Design review of the part built by this model. Coordinates are the model's own, in mm. Face numbers are marked on the shaded views. Coordinates: 2 decimals unless noted, no trailing zeros. Loops run counter-clockwise (first coordinate to the right, second up) from the corner with the lowest first, then second, coordinate; pieces in that order, holes last. Notation, with made-up numbers: (34.25, 73) - (69.25, 73) arc R24 ccw to (69.25, 83) - close; hole circle Ø5 at (48, 74.5). An arc over 180 degrees is marked (long way). One line per question, with ' | ' between items.
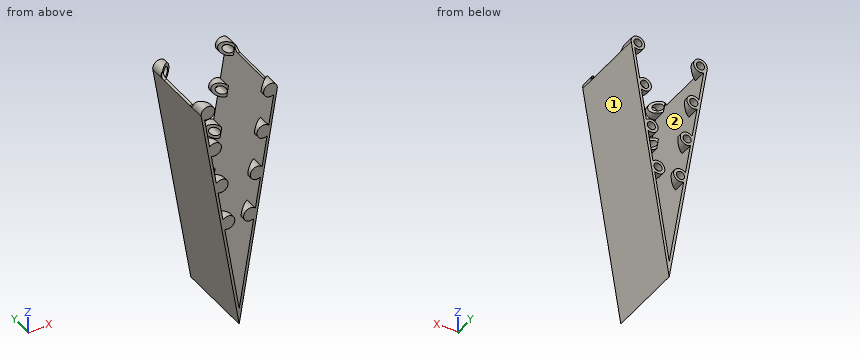
from build123d import *

# Parameters (mm, degrees)
BOSS_EXTRUDE1_DEPTH            = 30
SKETCH2_R                      = 2.6
SKETCH2_R_2                    = 1.55
BOSS_EXTRUDE3_DEPTH            = 5
CUT_EXTRUDE1_REACH             = 100.017
CUT_EXTRUDE1_DIRECTION_2_DEPTH = 99.016911981
CUT_EXTRUDE2_REACH             = 100.017
CUT_EXTRUDE2_DIRECTION_2_DEPTH = 99.016911981
FILLET1_R                      = 2
SKETCH6_R                      = 2.6
BOSS_EXTRUDE4_DEPTH            = 1


with BuildPart() as part:
    # Sketch1 → Boss-Extrude1 (new body)
    with BuildSketch(Plane(origin=(0, 0, 0), x_dir=(1, 0, 0), z_dir=(0, 1, 0))):
        Polygon((-13.5, 0), (0, 83.718518379), (13.5, 0), (14.487246657, 0.15919811), (0, 90), (-14.487246657, 0.15919811), align=None)
    extrude(amount=BOSS_EXTRUDE1_DEPTH)

    # Sketch2 → Boss-Extrude3 (add)
    # profile 1 of 8: a face of its own
    with BuildSketch(Plane(origin=(0, 0, 0), x_dir=(1, 0, 0), z_dir=(0, 1, 0))):
        with Locations((11.920405349, -0.254716975)):
            Circle(SKETCH2_R)
        with Locations(Location((11.920405349, -0.254716975, 0), (0, 0, 270))):
            Circle(SKETCH2_R_2, mode=Mode.SUBTRACT)
    # profile 2 of 8: a face of its own
    with BuildSketch(Plane(origin=(0, 0, 0), x_dir=(1, 0, 0), z_dir=(0, 1, 0))):
        with Locations((9.373235594, 15.541229537)):
            Circle(SKETCH2_R)
        with Locations(Location((9.373235594, 15.541229537, 0), (0, 0, 270))):
            Circle(SKETCH2_R_2, mode=Mode.SUBTRACT)
    # profile 3 of 8: a face of its own
    with BuildSketch(Plane(origin=(0, 0, 0), x_dir=(1, 0, 0), z_dir=(0, 1, 0))):
        with Locations((6.826065839, 31.33717605)):
            Circle(SKETCH2_R)
        with Locations(Location((6.826065839, 31.33717605, 0), (0, 0, 270))):
            Circle(SKETCH2_R_2, mode=Mode.SUBTRACT)
    # profile 4 of 8: a face of its own
    with BuildSketch(Plane(origin=(0, 0, 0), x_dir=(1, 0, 0), z_dir=(0, 1, 0))):
        with Locations((4.278896085, 47.133122563)):
            Circle(SKETCH2_R)
        with Locations(Location((4.278896085, 47.133122563, 0), (0, 0, 270))):
            Circle(SKETCH2_R_2, mode=Mode.SUBTRACT)
    # profile 5 of 8: a face of its own
    with BuildSketch(Plane(origin=(0, 0, 0), x_dir=(1, 0, 0), z_dir=(0, 1, 0))):
        with Locations((-4.278896085, 47.133122563)):
            Circle(SKETCH2_R)
        with Locations(Location((-4.278896085, 47.133122563, 0), (0, 0, 90))):
            Circle(SKETCH2_R_2, mode=Mode.SUBTRACT)
    # profile 6 of 8: a face of its own
    with BuildSketch(Plane(origin=(0, 0, 0), x_dir=(1, 0, 0), z_dir=(0, 1, 0))):
        with Locations((-6.826065839, 31.33717605)):
            Circle(SKETCH2_R)
        with Locations(Location((-6.826065839, 31.33717605, 0), (0, 0, 90))):
            Circle(SKETCH2_R_2, mode=Mode.SUBTRACT)
    # profile 7 of 8: a face of its own
    with BuildSketch(Plane(origin=(0, 0, 0), x_dir=(1, 0, 0), z_dir=(0, 1, 0))):
        with Locations((-9.373235594, 15.541229537)):
            Circle(SKETCH2_R)
        with Locations(Location((-9.373235594, 15.541229537, 0), (0, 0, 90))):
            Circle(SKETCH2_R_2, mode=Mode.SUBTRACT)
    # profile 8 of 8: a face of its own
    with BuildSketch(Plane(origin=(0, 0, 0), x_dir=(1, 0, 0), z_dir=(0, 1, 0))):
        with Locations((-11.920405349, -0.254716975)):
            Circle(SKETCH2_R)
        with Locations(Location((-11.920405349, -0.254716975, 0), (0, 0, 90))):
            Circle(SKETCH2_R_2, mode=Mode.SUBTRACT)
    boss_extrude3 = extrude(amount=BOSS_EXTRUDE3_DEPTH)

    # Cut-Extrude1: up to this face of the body (flat: up to its plane)
    cut_extrude1_end = Plane(part.part.faces().sort_by_distance((-6.68152525, 15.362665762, -42.28389657))[0])
    # Sketch4 → Cut-Extrude1 (cut, up to the picked face)
    with BuildSketch(Plane(origin=(0.342144515, 0, 2.121765321), x_dir=(0.9872466570606503, 0, -0.1591981096702188), z_dir=(0.1591981096702188, 0, 0.9872466570606503)), mode=Mode.PRIVATE) as cut_extrude1_sk1:
        Polygon((13.32782987, 5), (9.12782987, 5), (9.12782987, 1.475781549), align=None)
    cut_extrude1_tool1 = split(extrude(cut_extrude1_sk1.sketch, amount=-CUT_EXTRUDE1_REACH, mode=Mode.PRIVATE), bisect_by=cut_extrude1_end, keep=Keep.BOTH, mode=Mode.PRIVATE)
    cut_extrude1 = cut_extrude1_tool1.solids().sort_by(Axis((10.735709, 3.825261, 0.445755), (-0.1591981096702188, 0, -0.9872466570606503)))[0]
    add(cut_extrude1, mode=Mode.SUBTRACT)

    # Sketch4 → Cut-Extrude1 direction 2 (cut)
    with BuildSketch(Plane(origin=(0.342144515, 0, 2.121765321), x_dir=(0.9872466570606503, 0, -0.1591981096702188), z_dir=(0.1591981096702188, 0, 0.9872466570606503))):
        Polygon((13.32782987, 5), (9.12782987, 5), (9.12782987, 1.475781549), align=None)
    cut_extrude1_direction_2 = extrude(amount=CUT_EXTRUDE1_DIRECTION_2_DEPTH, mode=Mode.SUBTRACT)

    # Cut-Extrude2: up to this face of the body (flat: up to its plane)
    cut_extrude2_end = Plane(part.part.faces().sort_by_distance((6.68152525, 15.362665762, -42.28389657))[0])
    # Sketch5 → Cut-Extrude2 (cut, up to the picked face)
    with BuildSketch(Plane(origin=(-0.342144515, 0, 2.121765321), x_dir=(0.9872466570606502, 0, 0.15919810967021986), z_dir=(-0.15919810967021986, 0, 0.9872466570606502)), mode=Mode.PRIVATE) as cut_extrude2_sk1:
        Polygon((-9.12782987, 5), (-9.12782987, 1.475781549), (-13.32782987, 5), align=None)
    cut_extrude2_tool1 = split(extrude(cut_extrude2_sk1.sketch, amount=-CUT_EXTRUDE2_REACH, mode=Mode.PRIVATE), bisect_by=cut_extrude2_end, keep=Keep.BOTH, mode=Mode.PRIVATE)
    cut_extrude2 = cut_extrude2_tool1.solids().sort_by(Axis((-10.735709, 3.825261, 0.445755), (0.15919810967021986, 0, -0.9872466570606502)))[0]
    add(cut_extrude2, mode=Mode.SUBTRACT)

    # Sketch5 → Cut-Extrude2 direction 2 (cut)
    with BuildSketch(Plane(origin=(-0.342144515, 0, 2.121765321), x_dir=(0.9872466570606502, 0, 0.15919810967021986), z_dir=(-0.15919810967021986, 0, 0.9872466570606502))):
        Polygon((-9.12782987, 5), (-9.12782987, 1.475781549), (-13.32782987, 5), align=None)
    cut_extrude2_direction_2 = extrude(amount=CUT_EXTRUDE2_DIRECTION_2_DEPTH, mode=Mode.SUBTRACT)

    # Mirror2: Boss-Extrude3, Cut-Extrude1, Cut-Extrude1 direction 2, Cut-Extrude2, Cut-Extrude2 direction 2 across plane
    add(boss_extrude3.mirror(Plane.ZX.offset(15)))
    add(cut_extrude1.mirror(Plane.ZX.offset(15)), mode=Mode.SUBTRACT)
    add(cut_extrude1_direction_2.mirror(Plane.ZX.offset(15)), mode=Mode.SUBTRACT)
    add(cut_extrude2.mirror(Plane.ZX.offset(15)), mode=Mode.SUBTRACT)
    add(cut_extrude2_direction_2.mirror(Plane.ZX.offset(15)), mode=Mode.SUBTRACT)

    # Fillet1
    # the kernel refuses this fillet: 2 mm, written as the material it adds along each edge
    with BuildSketch(Plane(origin=(-19.423479942, 5, -0.955188658), x_dir=(-0.15919810967021975, 0, 0.9872466570606501), z_dir=(0.9872466570606501, 0, 0.15919810967021975))) as fillet1_piece_1_section:
        with BuildLine():
            CenterArc((FILLET1_R, -FILLET1_R), FILLET1_R, 90, 90)
            Line((0, -FILLET1_R), (0, 0))
            Line((0, 0), (FILLET1_R, 0))
        make_face()
    fillet1_piece_1 = extrude(amount=6, mode=Mode.PRIVATE)
    fillet1_piece_1 = fillet1_piece_1 & Plane(origin=(-11.920405349, 5.222362792, 0.254716975), x_dir=(1, 0, 0), z_dir=(0, -1, 0)) * Cylinder(2.6, 21, mode=Mode.PRIVATE)
    add(fillet1_piece_1)
    with BuildSketch(Plane(origin=(13.5, 5, 0), x_dir=(0, 1, 0), z_dir=(0.9872466570606502, 0, -0.15919810967021866))) as fillet1_piece_2_section:
        with BuildLine():
            CenterArc((FILLET1_R, FILLET1_R), FILLET1_R, 180, 90)
            Line((0, FILLET1_R), (0, 0))
            Line((0, 0), (FILLET1_R, 0))
        make_face()
    fillet1_piece_2 = extrude(amount=6, mode=Mode.PRIVATE)
    fillet1_piece_2 = fillet1_piece_2 & Plane(origin=(11.920405349, 5.699977741, 0.254716975), x_dir=(1, 0, 0), z_dir=(0, -1, 0)) * Cylinder(2.6, 20, mode=Mode.PRIVATE)
    add(fillet1_piece_2)
    with BuildSketch(Plane(origin=(13.5, 25, 0), x_dir=(0, -1, 0), z_dir=(0.9872466570606502, 0, -0.15919810967021866))) as fillet1_piece_3_section:
        with BuildLine():
            CenterArc((FILLET1_R, -FILLET1_R), FILLET1_R, 90, 90)
            Line((0, -FILLET1_R), (0, 0))
            Line((0, 0), (FILLET1_R, 0))
        make_face()
    fillet1_piece_3 = extrude(amount=6, mode=Mode.PRIVATE)
    fillet1_piece_3 = fillet1_piece_3 & Plane(origin=(11.920405349, 24.300022259, 0.254716975), x_dir=(1, 0, 0), z_dir=(0, 1, 0)) * Cylinder(2.6, 20, mode=Mode.PRIVATE)
    add(fillet1_piece_3)
    with BuildSketch(Plane(origin=(-19.423479942, 25, -0.955188658), x_dir=(0, -1, 0), z_dir=(0.9872466570606501, 0, 0.15919810967021975))) as fillet1_piece_4_section:
        with BuildLine():
            CenterArc((FILLET1_R, -FILLET1_R), FILLET1_R, 90, 90)
            Line((0, -FILLET1_R), (0, 0))
            Line((0, 0), (FILLET1_R, 0))
        make_face()
    fillet1_piece_4 = extrude(amount=6, mode=Mode.PRIVATE)
    fillet1_piece_4 = fillet1_piece_4 & Plane(origin=(-11.920405349, 24.777637105, 0.254716975), x_dir=(1, 0, 0), z_dir=(0, 1, 0)) * Cylinder(2.6, 21, mode=Mode.PRIVATE)
    add(fillet1_piece_4)

    # Sketch6 → Boss-Extrude4 (add)
    with BuildSketch(Plane.XZ):
        with Locations((11.920405349, 0.254716975)):
            Circle(SKETCH6_R)
        with Locations((9.373235594, -15.541229537)):
            Circle(SKETCH6_R)
        with Locations((6.826065839, -31.33717605)):
            Circle(SKETCH6_R)
        with Locations((4.278896085, -47.133122563)):
            Circle(SKETCH6_R)
        with Locations((-4.278896085, -47.133122563)):
            Circle(SKETCH6_R)
        with Locations((-6.826065839, -31.33717605)):
            Circle(SKETCH6_R)
        with Locations((-9.373235594, -15.541229537)):
            Circle(SKETCH6_R)
        with Locations((-11.920405349, 0.254716975)):
            Circle(SKETCH6_R)
    extrude(amount=-BOSS_EXTRUDE4_DEPTH)


solid = part.part
Q1. For pin 1 (1.5 mm diameter, centred on y = 16.5, z = -31.5, fed in from -X); pin 2 (10 mm diameter, centred on x = -9.5, z = -67.5, fed in from +Y); pin 3 (3 mm diameter, centred on y = 26.5, z = -49.5, fed in from -X), all flat-tipped, find the tip position at first contact; note any pin that passes through.
Returned:
pin 1: stops at x = -9.55 | pin 2: passes through | pin 3: stops at x = -6.77
Q2. Take a section at A-A (z = -40). Give the boundary of the cut face in (x, y).
Returned:
outline: (-8.06, 0) - (-7.05, 0) - (-7.05, 30) - (-8.06, 30) - close; (7.05, 0) - (8.06, 0) - (8.06, 30) - (7.05, 30) - close
Q3. Take a section at B-B (y = 10). Give the boundary of the cut face in (x, z).
Returned:
outline: (-14.49, -0.16) - (0, -90) - (14.49, -0.16) - (13.5, 0) - (0, -83.72) - (-13.5, 0) - close
Q4. To check wall thickness, follow line 1 along Y through (x, z) = (-4, -46.5); line 2 along Y through (x, z) = (2.5, -48); line 3 along X through (y, z) = (18, -62.5). State the ranges of each line that lie inside material, in increasing order.
Returned:
line 1: y = 0 to 1 | line 2: y = 0 to 2.3, 27.7 to 30 | line 3: x = -4.43 to -3.42, 3.42 to 4.43
Q5. Draft analysis for pull direction Z (two halves, no side actions). For the marked faces 1 and 2, state which applies: +Z half, -Z half, draft (parallel to the pull), parting line (faces both ways), or undercut.
Returned:
face 1: -Z half | face 2: undercut
